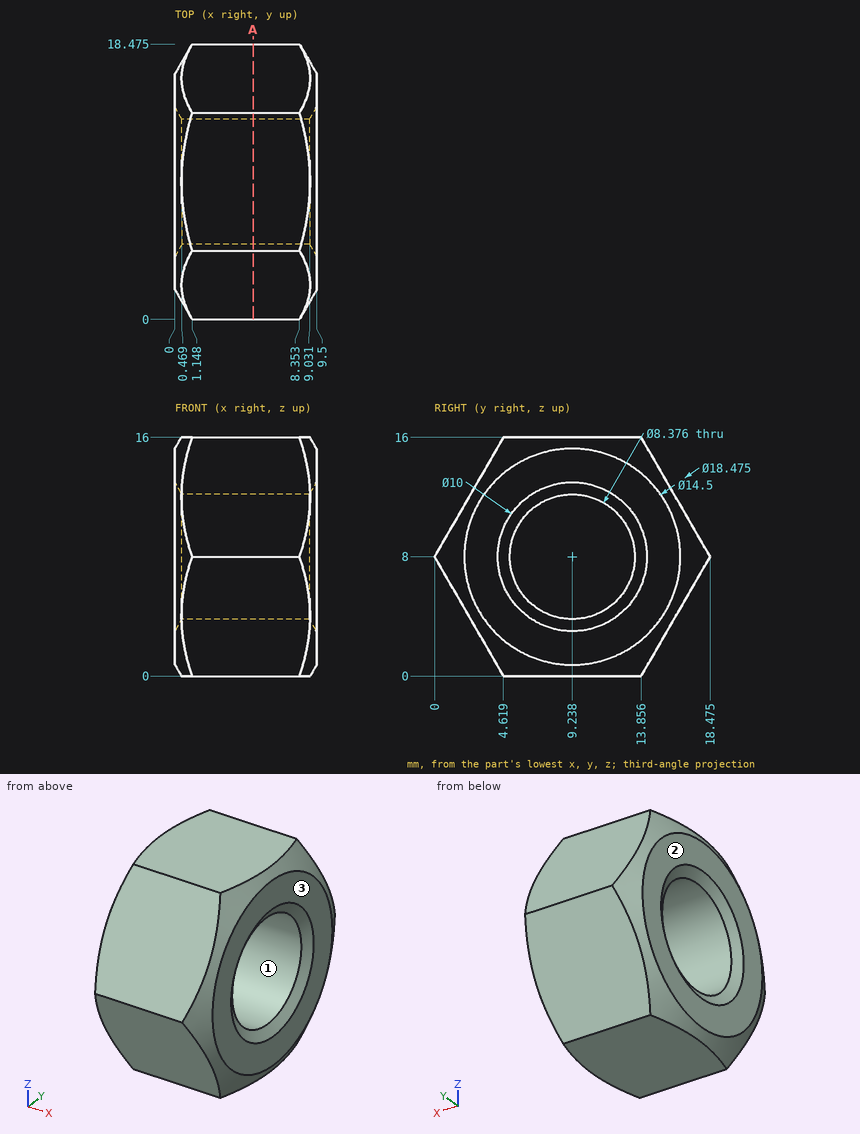
Part print with two shaded views. Sizes in mm from the minimum x, y, z corner. Coordinates: 2 decimals unless noted, no trailing zeros. Write each loop counter-clockwise with the first axis right and the second up, starting at its lowest first coordinate (ties: lowest second). Pieces come first, ordered by that corner, then holes. Notation, with made-up numbers: (34, 0.5) - (58, 0.5) arc R27 ccw to (58, 36.5) - close; hole circle Ø5 at (22, 49.5). An arc over 180 degrees is marked (long way). Use a Markdown table: item, result. Add a question column.
Item 1: Drill centre lines: line 1 along Y through (x, z) = (8, 11) (1 decimal); line 2 along Y through (x, z) = (6.5, 9.75) (1 decimal); line 3 along Z through (x, y) = (8.5, 12.25). Where is each one in solid material? Low to high.
Item 2: Band-saw the part on A-A, the plane x = 5.25. Write the cut outline in (y, z) (1 decimal), and give its area (3 significant figures).
Item 3: Drop flat-ended pins along their axis: pin 1 (5 mm diameter, centred on x = 7.5, y = 2, fed in from -Z) (1 decimal); pin 2 (4 mm diameter, centred on y = 3.5, z = 13, fed in from -X); pin 3 (9.5 mm diameter, centred on y = 9.24, z = 8, fed in from -X); pin 4 (1 mm diameter, centred on x = 8, z = 10.5, fed in from -Y) (1 decimal). Give the stop position or say it passes through.
Item 4: Two-plate mould, pull along X, no slides. Class the marked faces 1, 2 and 3: pulls with the +X half, pulls with the -X half, needs draft (parallel to the pull), parting line crosses it, or undercut.
A:
| question | item | result |
|---|---|---|
| 1 | line 1 | y = 1.7 to 6.3, 12.2 to 16.7 |
| 1 | line 2 | y = 1 to 5.4, 13 to 17.5 |
| 1 | line 3 | z = 0 to 5.09, 10.91 to 16 |
| 2 | outline | (0, 8) - (4.6, 0) - (13.9, 0) - (18.5, 8) - (13.9, 16) - (4.6, 16) - close; hole circle Ø8.4 at (9.2, 8) |
| 2 | area | 167 mm² |
| 3 | pin 1 | stops at z = 0.2 |
| 3 | pin 2 | stops at x = 0 |
| 3 | pin 3 | stops at x = 0.14 |
| 3 | pin 4 | stops at y = 1.2 |
| 4 | face 1 | needs draft |
| 4 | face 2 | pulls with the -X half |
| 4 | face 3 | pulls with the +X half |
